```python
from build123d import *

# Parameters (mm, degrees)
CROQUIS1_R              = 3.2
SALIENTE_EXTRUIR1_DEPTH = 0.75
SALIENTE_EXTRUIR2_START = 3.5
CROQUIS2_R              = 6
CROQUIS2_R_2            = 3.2
SALIENTE_EXTRUIR2_DEPTH = 3.5


with BuildPart() as part:
    # Croquis1 → Saliente-Extruir1 (new, symmetric)
    # profile 1 of 9: a face of its own
    with BuildSketch(Plane(origin=(0, 0, 0), x_dir=(0, 0, -1), z_dir=(1, 0, 0))):
        with BuildLine():
            ThreePointArc((-2.2961005941905754, 5.543277195067705), (-1.1705419320967896, 5.884711682419379), (0, 5.999999999999999))
            Line((0, 6), (0, 15))
            ThreePointArc((9.2e-16, 14.999999999999998), (-2.9263548302419715, 14.711779206048444), (-5.740251485476437, 13.85819298766926))
            Line((-5.740251485476437, 13.858192987669263), (-2.296100594190576, 5.543277195067706))
        make_face()
    # profile 2 of 9: a face of its own
    with BuildSketch(Plane(origin=(0, 0, 0), x_dir=(0, 0, -1), z_dir=(1, 0, 0))):
        with BuildLine():
            Line((0, 15), (0, 6))
            ThreePointArc((3.7e-16, 6), (1.1705419320967503, 5.884711682419386), (2.296100594190503, 5.543277195067735))
            Line((2.2961005941905026, 5.543277195067734), (5.740251485476257, 13.858192987669337))
            ThreePointArc((5.740251485476257, 13.858192987669337), (2.9263548302418774, 14.711779206048465), (1.1e-16, 15))
        make_face()
    # profile 3 of 9: a face of its own
    with BuildSketch(Plane(origin=(0, 0, 0), x_dir=(0, 0, -1), z_dir=(1, 0, 0))):
        with BuildLine():
            Line((13.858192987669264, 5.740251485476436), (5.543277195067706, 2.296100594190575))
            ThreePointArc((5.543277195067704, 2.2961005941905754), (5.884711682419379, 1.1705419320967891), (6, 3.7e-16))
            Line((6, 3.7e-16), (15, 9.2e-16))
            ThreePointArc((14.999999999999998, 0), (14.711779206048446, 2.9263548302419706), (13.858192987669263, 5.740251485476435))
        make_face()
    # profile 4 of 9: a face of its own
    with BuildSketch(Plane(origin=(0, 0, 0), x_dir=(0, 0, -1), z_dir=(1, 0, 0))):
        with BuildLine():
            Line((15, 9.2e-16), (6, 3.7e-16))
            ThreePointArc((6, -1.47e-15), (5.884711682419386, -1.1705419320967514), (5.543277195067735, -2.296100594190503))
            Line((5.543277195067734, -2.296100594190502), (13.858192987669337, -5.740251485476256))
            ThreePointArc((13.858192987669337, -5.740251485476256), (14.711779206048465, -2.9263548302418743), (14.999999999999998, 1.11e-15))
        make_face()
    # profile 5 of 9: a face of its own
    with BuildSketch(Plane(origin=(0, 0, 0), x_dir=(0, 0, -1), z_dir=(1, 0, 0))):
        with BuildLine():
            Line((5.740251485476437, -13.858192987669264), (2.2961005941905754, -5.543277195067704))
            ThreePointArc((2.296100594190576, -5.543277195067706), (1.17054193209679, -5.88471168241938), (9.2e-16, -6.000000000000001))
            Line((9.2e-16, -6), (1.84e-15, -15))
            ThreePointArc((-2.76e-15, -14.999999999999998), (2.9263548302419635, -14.711779206048446), (5.740251485476435, -13.858192987669263))
        make_face()
    # profile 6 of 9: a face of its own
    with BuildSketch(Plane(origin=(0, 0, 0), x_dir=(0, 0, -1), z_dir=(1, 0, 0))):
        with BuildLine():
            ThreePointArc((-1.1e-15, -6), (-1.170541932096751, -5.884711682419386), (-2.2961005941905026, -5.543277195067736))
            Line((-2.2961005941905017, -5.543277195067734), (-5.740251485476255, -13.858192987669337))
            ThreePointArc((-5.740251485476255, -13.858192987669337), (-2.9263548302418756, -14.711779206048465), (1.67e-15, -15))
            Line((1.84e-15, -15), (9.2e-16, -6))
        make_face()
    # profile 7 of 9: a face of its own
    with BuildSketch(Plane(origin=(0, 0, 0), x_dir=(0, 0, -1), z_dir=(1, 0, 0))):
        with BuildLine():
            ThreePointArc((-5.543277195067704, -2.296100594190576), (-5.884711682419379, -1.17054193209679), (-6, -1.1e-15))
            Line((-6, -1.1e-15), (-15, -2.76e-15))
            ThreePointArc((-14.999999999999998, 1.84e-15), (-14.711779206048446, -2.9263548302419706), (-13.858192987669263, -5.740251485476436))
            Line((-13.858192987669264, -5.740251485476437), (-5.543277195067706, -2.296100594190576))
        make_face()
    # profile 8 of 9: a face of its own
    with BuildSketch(Plane(origin=(0, 0, 0), x_dir=(0, 0, -1), z_dir=(1, 0, 0))):
        with BuildLine():
            ThreePointArc((-6, 7.3e-16), (-5.884711682419386, 1.1705419320967507), (-5.543277195067736, 2.296100594190502))
            Line((-5.543277195067736, 2.296100594190502), (-13.858192987669339, 5.7402514854762545))
            ThreePointArc((-13.85819298766934, 5.740251485476255), (-14.711779206048467, 2.9263548302418747), (-15.000000000000002, -3.22e-15))
            Line((-15, -2.76e-15), (-6, -1.1e-15))
        make_face()
    # profile 9 of 9: a face of its own
    with BuildSketch(Plane(origin=(0, 0, 0), x_dir=(0, 0, -1), z_dir=(1, 0, 0))):
        with BuildLine():
            ThreePointArc((2.296100594190503, 5.543277195067735), (1.1705419320967503, 5.884711682419386), (3.7e-16, 6))
            ThreePointArc((0, 5.999999999999999), (-1.1705419320967896, 5.884711682419379), (-2.2961005941905754, 5.543277195067705))
            ThreePointArc((-2.2961005941905763, 5.543277195067705), (-3.3334213981176317, 4.98881767381526), (-4.2426406871192865, 4.242640687119284))
            ThreePointArc((-4.242640687119286, 4.242640687119283), (-4.988817673815284, 3.333421398117596), (-5.543277195067734, 2.2961005941905004))
            ThreePointArc((-5.543277195067736, 2.296100594190502), (-5.884711682419386, 1.1705419320967507), (-6, 7.3e-16))
            ThreePointArc((-6, -1.1e-15), (-5.884711682419379, -1.17054193209679), (-5.543277195067704, -2.296100594190576))
            ThreePointArc((-5.543277195067706, -2.2961005941905746), (-4.9888176738152605, -3.333421398117629), (-4.242640687119286, -4.242640687119285))
            ThreePointArc((-4.242640687119285, -4.242640687119287), (-3.333421398117597, -4.988817673815285), (-2.2961005941905013, -5.543277195067736))
            ThreePointArc((-2.2961005941905026, -5.543277195067736), (-1.170541932096751, -5.884711682419386), (-1.1e-15, -6))
            ThreePointArc((9.2e-16, -6.000000000000001), (1.17054193209679, -5.88471168241938), (2.296100594190576, -5.543277195067706))
            ThreePointArc((2.296100594190574, -5.543277195067706), (3.333421398117629, -4.9888176738152605), (4.242640687119284, -4.242640687119286))
            ThreePointArc((4.2426406871192865, -4.242640687119285), (4.988817673815282, -3.333421398117596), (5.543277195067736, -2.296100594190502))
            ThreePointArc((5.543277195067735, -2.296100594190503), (5.884711682419386, -1.1705419320967514), (6, -1.47e-15))
            ThreePointArc((6, 3.7e-16), (5.884711682419379, 1.1705419320967891), (5.543277195067704, 2.2961005941905754))
            ThreePointArc((5.543277195067705, 2.2961005941905754), (4.9888176738152605, 3.333421398117629), (4.242640687119286, 4.242640687119284))
            ThreePointArc((4.242640687119287, 4.2426406871192865), (3.333421398117599, 4.988817673815284), (2.2961005941905035, 5.543277195067736))
        make_face()
        Circle(CROQUIS1_R, mode=Mode.SUBTRACT)
    extrude(amount=SALIENTE_EXTRUIR1_DEPTH, both=True)

    # Croquis2 → Saliente-Extruir2 (add)
    with BuildSketch(Plane(origin=(0.75, 0, 0), x_dir=(0, 0, -1), z_dir=(1, 0, 0)).offset(SALIENTE_EXTRUIR2_START)):
        with Locations(Location((0, 0, 0), (0, 0, 157.5))):
            Circle(CROQUIS2_R)
        Circle(CROQUIS2_R_2, mode=Mode.SUBTRACT)
    extrude(amount=-SALIENTE_EXTRUIR2_DEPTH)


solid = part.part
```
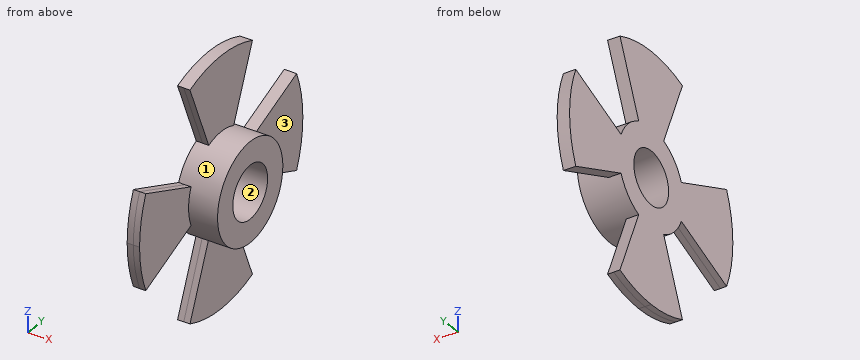
Here's how the part is built. I have some questions about the finished solid (model axes, mm). Face numbers are marked on the shaded views. Give positions to 0.01 mm unless a question says otherwise; leave off trailing zeros. Order: outer loops, then holes, each group sorted by start corner. A loop starts at its lowest first (then second) coordinate and runs counter-clockwise, first axis right, second up. Notation, with made-up numbers: (5.25, 32.25) -> (15.25, 32.25) arc R10 cw to (15.25, 43.25) -> close; hole circle Ø8 at (85, 44). An arc over 180 degrees is marked (long way). Use CSV: the item, a comma, the result in double quotes. Start each with the question number.
Item 1: Thinking about a two-plate mould opening in Z: for the marked faces 1, 2 and 3, which applies, pulls with the +Z half, pulls with the -Z half, needs draft (parallel to the pull), parting line crosses it, or undercut?
Item 2: If I drill on probe 1 along Y at (x, z) = (3.15, 0); probe 2 along Y at (x, z) = (0.5, 0); probe 3 along X at (y, z) = (12.25, 3), over which ranges is the centre line in solid material (lowest first)? Write a range as [from, to].
Item 3: Suppose I cut it at D-D (y = 4). List the corners of the cut face in (x, z) for me, and give its area (3 significant figures).
Item 4: I'm going to push flat-ended pins straight in: P1, Ø4.5, axis at y = 0.5, z = -11.5, coming from the +X side; P2, Ø1.5, axis at x = 0.5, z = 10, coming from the +Y side. Where does each tip first touch, or does it pass through?
Item 5: Suppose I cut it at A-A (z = 0.5). List the corners of the cut face in (x, y) for me, and give its area (3 significant figures).
Item 6: Suppose I cut it at C-C (x = 2.85). List the corners of the cut face in (y, z) for me.
Answer block:
1,face 1,"undercut"
1,face 2,"undercut"
1,face 3,"needs draft"
2,probe 1,"y = [-6, -3.2], [3.2, 6]"
2,probe 2,"y = [-15, -3.2], [3.2, 15]"
2,probe 3,"x = [-0.75, 0.75]"
3,outline,"(-0.75, -14.46) -> (0.75, -14.46) -> (0.75, -9.66) -> (-0.75, -9.66) -> close; (-0.75, -4.47) -> (4.25, -4.47) -> (4.25, 4.47) -> (-0.75, 4.47) -> close; (-0.75, 9.66) -> (0.75, 9.66) -> (0.75, 14.46) -> (-0.75, 14.46) -> close"
3,area,"59.1 mm^2"
4,P1,"stops at x = 0.75"
4,P2,"stops at y = 4.45"
5,outline,"(-0.75, -14.99) -> (0.75, -14.99) -> (0.75, -5.98) -> (4.25, -5.98) -> (4.25, -3.16) -> (-0.75, -3.16) -> close; (-0.75, 3.16) -> (4.25, 3.16) -> (4.25, 5.98) -> (0.75, 5.98) -> (0.75, 14.99) -> (-0.75, 14.99) -> close"
5,area,"55.2 mm^2"
6,outline,"circle Ø12 at (0, 0); hole circle Ø6.4 at (0, 0)"
